Design review of the part built by this model. Coordinates are the model's own, in mm. Face numbers are marked on the shaded views. A direction names the side the tool comes from. Coordinates: 2 decimals unless noted, no trailing zeros. Loops run counter-clockwise (first coordinate to the right, second up) from the corner with the lowest first, then second, coordinate; pieces in that order, holes last. Notation, with made-up numbers: (-11.5, 3) -> (30.5, 3) arc R24 ccw to (30.5, 17) -> close; hole circle Ø6 at (67.5, -36.5). An arc over 180 degrees is marked (long way). One line per item, written item: value. Start each with the question number.
1. Add section C-C on x = 0. Write out the cut boundary in (y, z).
2. Machinability: for the marked faces 5 and 6, which of the approach directions +Z, -Z, +X, -X, +Y, -Y give a long, thin tool a straight path to every point of the face, cutting with its end or side? Answer none if there is none.
3. Add section A-A on y = 0. Write out the cut boundary in (x, z).
4. Insertion check: pin 1 (5 mm diameter, centred on y = -5, z = 7.5, fed in from -X); pin 2 (4 mm diameter, centred on x = 1.5, y = 0, fed in from +Z); pin 3 (1 mm diameter, centred on y = -2, z = -8, fed in from -X). Each pin has a flat end and moves straight along its axis. Give the tip position at first contact, or say it passes through.
5. For probe 1 along Z at (x, y) = (0, -4.95); probe 2 along Z at (x, y) = (-1.75, -6); probe 3 along Z at (x, y) = (0, -3.25), list the stretches that pass through material, from the lowest coordinate up.
6. Add section D-D on y = -3. Write out the cut boundary in (x, z).
7. Add section B-B on z = 6.25. Write out the cut boundary in (x, y).
8. Draft analysis for pull direction Z (two halves, no side actions). For the marked faces 1, 2, 3 and 4, state which applies: pulls with the +Z half, pulls with the -Z half, needs draft (parallel to the pull), parting line crosses it, or undercut.
Autodesk Fusion 360 part; units mm, degrees
sketch "Sketch1" plane through (0, 0, 0) normal (0, 0, 1) x (1, 0, 0)
  circle A0 centre (0, 0) radius 2.5
  circle A1 centre (0, 0) radius 4
  circle A2 centre (0, 0) radius 7
  dimension "d1" = 5
  dimension "d2" = 8
  dimension "d3" = 14
extrude "Extrude1" add sketch "Sketch1" along normal blind 12.5 contours A2
extrude "Extrude2" add sketch "Sketch1" against normal blind 12.5 contours A1 | A2
sketch "Sketch2" plane through (0, 0, 0) normal (0, 1, 0) x (1, 0, 0)
  line L0 (7, 12.5) -> (-7, 12.5)
  line L1 (-7, -12.5) -> (7, -12.5)
  line L2 (0, 12.5) -> (0, 6.25)
  circle A0 centre (0, 6.25) radius 2.25
  line L3 (1.75, 0) -> (22.5, 0)
  circle A1 centre (0, -6.25) radius 2.25
  dimension "d8" = 6.25
  dimension "d9" = 4.5
extrude "Extrude3" cut sketch "Sketch2" along normal through all and the other way through all
thread "Thread1"
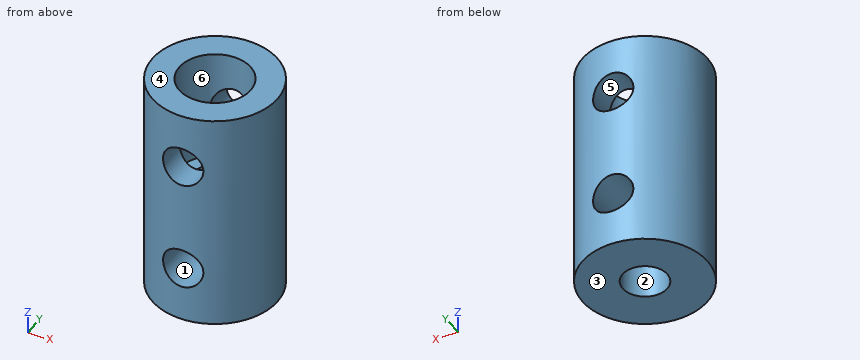
Worked answers:
1. outline: (-7, -12.5) -> (-2.5, -12.5) -> (-2.5, -8.5) -> (-7, -8.5) -> close; (-7, -4) -> (-2.5, -4) -> (-2.5, 0) -> (-4, 0) -> (-4, 4) -> (-7, 4) -> close; (-7, 8.5) -> (-4, 8.5) -> (-4, 12.5) -> (-7, 12.5) -> close; (2.5, -12.5) -> (7, -12.5) -> (7, -8.5) -> (2.5, -8.5) -> close; (2.5, -4) -> (7, -4) -> (7, 4) -> (4, 4) -> (4, 0) -> (2.5, 0) -> close; (4, 8.5) -> (7, 8.5) -> (7, 12.5) -> (4, 12.5) -> close
2. face 5: +Y, -Y
2. face 6: +Z
3. outline: (-7, -12.5) -> (-2.5, -12.5) -> (-2.5, 0) -> (-4, 0) -> (-4, 12.5) -> (-7, 12.5) -> close; (2.5, -12.5) -> (7, -12.5) -> (7, 12.5) -> (4, 12.5) -> (4, 0) -> (2.5, 0) -> close
4. pin 1: stops at x = -6.54
4. pin 2: stops at z = 0
4. pin 3: stops at x = -6.84
5. probe 1: z = -12.5 to -8.5, -4 to 4, 8.5 to 12.5
5. probe 2: z = -12.5 to -7.66, -4.84 to 4.84, 7.66 to 12.5
5. probe 3: z = -12.5 to -8.5, -4 to 0
6. outline: (-6.32, -12.5) -> (6.32, -12.5) -> (6.32, 12.5) -> (2.65, 12.5) -> (2.65, 0) -> (-2.65, 0) -> (-2.65, 12.5) -> (-6.32, 12.5) -> close; hole circle Ø4.5 at (0, -6.25)
7. outline: (-2.25, -6.63) -> (-2.25, -3.31) arc R4 cw to (-2.25, 3.31) -> (-2.25, 6.63) arc R7 ccw to start; (2.25, -6.63) arc R7 ccw to (2.25, 6.63) -> (2.25, 3.31) arc R4 cw to (2.25, -3.31) -> close
8. face 1: undercut
8. face 2: needs draft
8. face 3: pulls with the -Z half
8. face 4: pulls with the +Z half
